from build123d import *

# Parameters (mm, degrees)
F1_DEPTH = 28
F2_R     = 3
F3_T     = -2.5
F5_DEPTH = 25.5
F7_DEPTH = 2.5


with BuildPart() as f1:
    # F0 (on Top) → F1 (new body)
    with BuildSketch(Plane.XY):
        Polygon((-37.5, 27.5), (-37.5, -27.5), (37.5, -27.5), (37.5, 27.5), (20, 27.5), (20, 46.1637973785), (5, 46.1637973785), (5, 27.5), align=None)
    extrude(amount=F1_DEPTH)

    # F2
    f2_edges = [f1.edges().sort_by_distance(p)[0] for p in [
        (0, -27.5, 28),
        (37.5, 0, 28),
        (28.75, 27.5, 28),
        (37.5, 27.5, 14),
        (-37.5, 0, 28),
        (37.5, -27.5, 14),
        (-37.5, -27.5, 14),
        (-16.25, 27.5, 28),
        (5, 36.831899, 28),
        (5, 27.5, 14),
        (-37.5, 27.5, 14),
        (20, 27.5, 14),
        (20, 36.831899, 28),
    ]]
    fillet(f2_edges, radius=F2_R)

    # F3
    f3_openings = [f1.faces().sort_by_distance(p)[0] for p in [
        (0.806106, 2.36763, 0),
        (12.5, 46.163797, 13.876264),
    ]]
    offset(amount=F3_T, openings=f3_openings)

    # F4 (on Top) → F5 (join, through all)
    with BuildSketch(Plane.XY):
        Polygon((17.5, 12.5), (17.5, -25), (20, -25), (20, 10), (35, 10), (35, 12.5), align=None)
        Polygon((-12.5, 17.5), (-12.5, 25), (-15, 25), (-15, 20), (-35, 20), (-35, 17.5), align=None)
    extrude(amount=F5_DEPTH)

    # F6 (on face) → F7 (cut, through all)
    with BuildSketch(Plane.XY.offset(28)):
        Polygon((2.5, 12.5), (-2.5, 12.5), (-2.5, 2.5), (-12.5, 2.5), (-12.5, -2.5), (-2.5, -2.5), (-2.5, -12.5), (2.5, -12.5), (2.5, -2.5), (12.5, -2.5), (12.5, 2.5), (2.5, 2.5), align=None)
    extrude(amount=-F7_DEPTH, mode=Mode.SUBTRACT)


solid = f1.part
Source: CAD feature listing. Evaluate the final solid. Frame: model axes, mm. A direction names the side the tool comes from. Coordinates: 2 decimals unless noted, no trailing zeros. Loops run counter-clockwise (first coordinate to the right, second up) from the corner with the lowest first, then second, coordinate; pieces in that order, holes last. Notation, with made-up numbers: (29, 47.5) -> (65, 47.5) arc R15 ccw to (65, 69.5) -> close; hole circle Ø1 at (51.25, 44). An arc over 180 degrees is marked (long way). Answer in a Markdown table with one row per item. Add a question column.
Q1. Section C-C on y = -8. Return the cut outline in (x, z), and give its area (3 significant figures).
Q2. Reachability of faces 4 (the face through (27, -25, 12)), 5 (the face through (7.5, 38, 12)), 6 (the face through (-12.5, 0, 27)) from +Z, -Z, +X, -X, +Y, -Y: full face, straight path, thin tool, end or side. Return the list, or none.
Q3. Section A-A on y = 1.5. Return the cut outline in (x, z).
Q4. Ray query, line 1 along Y through (x, z) = (33, 5); line 2 along Y through (x, z) = (-33, 7.5); line 3 along X through (y, z) = (24, 11.75). Return the intervals inside material, ascending.
Q5. Contact query for flat-ended pins moving along their axis: pin 1 Ø1.2 at (x, z) = (-9, 26.5) entering from -Y; pin 2 Ø1 at (x, z) = (11.5, 4.5) entering from +Y; pin 3 Ø1 at (y, z) = (34, 5.5) entering from +X. Output: stop coordinate, or through.
Q6. Section B-B on x = -6. Return the cut outline in (y, z), and give its area (3 significant figures).
Q7. Section D-D on x = -30.5. Return the cut outline in (y, z), and give its area (3 significant figures).
Q8. Pull-direction query (X, two-part tool) for faces 1 (the face through (20.9, 28.36, 12.68)), 2 (the face through (-9, -25, 12)), 3 (the face through (-37.5, 0, 12)); classes: pulls with the +X half, pulls with the -X half, needs draft (parallel to the pull), parting line crosses it, or undercut.
Computed values:
| question | item | result |
|---|---|---|
| 1 | outline | (-37.5, 0) -> (-35, 0) -> (-35, 25) arc R0.5 cw to (-34.5, 25.5) -> (-2.5, 25.5) -> (-2.5, 28) -> (-34.5, 28) arc R3 ccw to (-37.5, 25) -> close; (2.5, 25.5) -> (17.5, 25.5) -> (17.5, 0) -> (20, 0) -> (20, 25.5) -> (34.5, 25.5) arc R0.5 cw to (35, 25) -> (35, 0) -> (37.5, 0) -> (37.5, 25) arc R3 ccw to (34.5, 28) -> (2.5, 28) -> close |
| 1 | area | 362 mm^2 |
| 2 | face 4 | -Z |
| 2 | face 5 | -Z, +Y |
| 2 | face 6 | +Z, -Z |
| 3 | outline | (-37.5, 0) -> (-35, 0) -> (-35, 25) arc R0.5 cw to (-34.5, 25.5) -> (-12.5, 25.5) -> (-12.5, 28) -> (-34.5, 28) arc R3 ccw to (-37.5, 25) -> close; (12.5, 25.5) -> (17.5, 25.5) -> (17.5, 0) -> (20, 0) -> (20, 25.5) -> (34.5, 25.5) arc R0.5 cw to (35, 25) -> (35, 0) -> (37.5, 0) -> (37.5, 25) arc R3 ccw to (34.5, 28) -> (12.5, 28) -> close |
| 4 | line 1 | y = -27.5 to -25, 10 to 12.5, 25 to 27.5 |
| 4 | line 2 | y = -27.5 to -25, 17.5 to 20, 25 to 27.5 |
| 4 | line 3 | x = -37.5 to -35, -15 to -12.5, 35 to 37.5 |
| 5 | pin 1 | stops at y = -27.36 |
| 5 | pin 2 | stops at y = -25 |
| 5 | pin 3 | stops at x = 20 |
| 6 | outline | (-27.5, 0) -> (-25, 0) -> (-25, 25) arc R0.5 cw to (-24.5, 25.5) -> (-2.5, 25.5) -> (-2.5, 28) -> (-24.5, 28) arc R3 ccw to (-27.5, 25) -> close; (2.5, 25.5) -> (24.5, 25.5) arc R0.5 cw to (25, 25) -> (25, 0) -> (27.5, 0) -> (27.5, 25) arc R3 ccw to (24.5, 28) -> (2.5, 28) -> close |
| 6 | area | 249 mm^2 |
| 7 | outline | (-27.5, 0) -> (-25, 0) -> (-25, 25) arc R0.5 cw to (-24.5, 25.5) -> (17.5, 25.5) -> (17.5, 0) -> (20, 0) -> (20, 25.5) -> (24.5, 25.5) arc R0.5 cw to (25, 25) -> (25, 0) -> (27.5, 0) -> (27.5, 25) arc R3 ccw to (24.5, 28) -> (-24.5, 28) arc R3 ccw to (-27.5, 25) -> close |
| 7 | area | 325 mm^2 |
| 8 | face 1 | pulls with the +X half |
| 8 | face 2 | undercut |
| 8 | face 3 | pulls with the -X half |
